from build123d import *

# Parameters (mm, degrees)
SKETCH1_W             = 50
SKETCH1_H             = 14
BOSS_EXTRUDE1_DEPTH   = 2.5
M4X0_7_TAPPED_HOLE1_D = 3.3


with BuildPart() as part:
    # Sketch1 → Boss-Extrude1 (new body, symmetric)
    with BuildSketch(Plane.XY):
        Rectangle(SKETCH1_W, SKETCH1_H)
    extrude(amount=BOSS_EXTRUDE1_DEPTH, both=True)

    # M4x0.7 Tapped Hole1 (through all)
    with Locations(Plane.XY.offset(2.5)):
        with Locations((-10, 0), (10, 0)):
            Hole(M4X0_7_TAPPED_HOLE1_D / 2)


solid = part.part
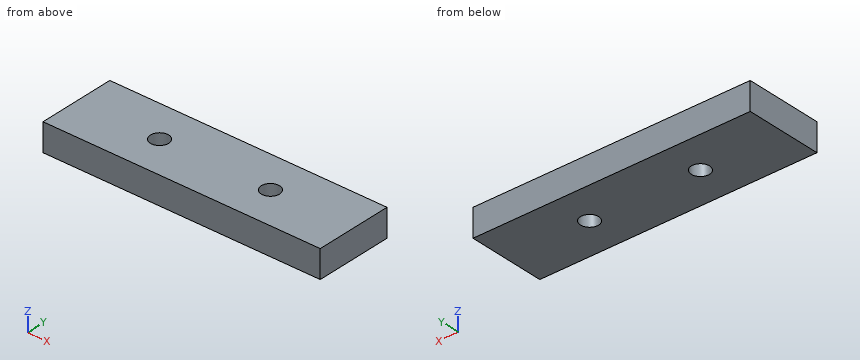
Model file for the job. Use its own axes, mm. Give positions to 0.01 mm unless a question says otherwise; leave off trailing zeros. Loops run counter-clockwise (first coordinate to the right, second up) from the corner with the lowest first, then second, coordinate; pieces in that order, holes last.
1) Saw through at B-B (x = -10). Write the cut outline in (y, z), plus the area to 3 significant figures.
2) Wall check: line 1 (Y direction, x = 10, z = 0.6); line 2 (X direction, y = 0.5, z = 0.45); line 3 (X direction, y = 1.5, z = -0.75). Give the ranges that are in metal, low to high.
3) Flat gauge pin, fed straight in: pin 1 Ø1.5 at (x, y) = (-10.5, -0.5) entering from -Z. Where does the tip first touch, or does it go through?
4) Saw through at A-A (y = 0). Write the cut outline in (x, z).
5) Saw through at D-D (x = 11). Write the cut outline in (y, z), plus the area to 3 significant figures.
6) Saw through at C-C (z = 1.65). Write the cut outline in (x, y), plus the area to 3 significant figures.
Answer block:
1. outline: (-7, -2.5) - (-1.65, -2.5) - (-1.65, 2.5) - (-7, 2.5) - close; (1.65, -2.5) - (7, -2.5) - (7, 2.5) - (1.65, 2.5) - close
1. area: 53.5 mm2
2. line 1: y = -7 to -1.65, 1.65 to 7
2. line 2: x = -25 to -11.57, -8.43 to 8.43, 11.57 to 25
2. line 3: x = -25 to -10.69, -9.31 to 9.31, 10.69 to 25
3. pin 1: passes through
4. outline: (-25, -2.5) - (-11.65, -2.5) - (-11.65, 2.5) - (-25, 2.5) - close; (-8.35, -2.5) - (8.35, -2.5) - (8.35, 2.5) - (-8.35, 2.5) - close; (11.65, -2.5) - (25, -2.5) - (25, 2.5) - (11.65, 2.5) - close
5. outline: (-7, -2.5) - (-1.31, -2.5) - (-1.31, 2.5) - (-7, 2.5) - close; (1.31, -2.5) - (7, -2.5) - (7, 2.5) - (1.31, 2.5) - close
5. area: 56.9 mm2
6. outline: (-25, -7) - (25, -7) - (25, 7) - (-25, 7) - close; hole circle Ø3.3 at (-10, 0); hole circle Ø3.3 at (10, 0)
6. area: 683 mm2
